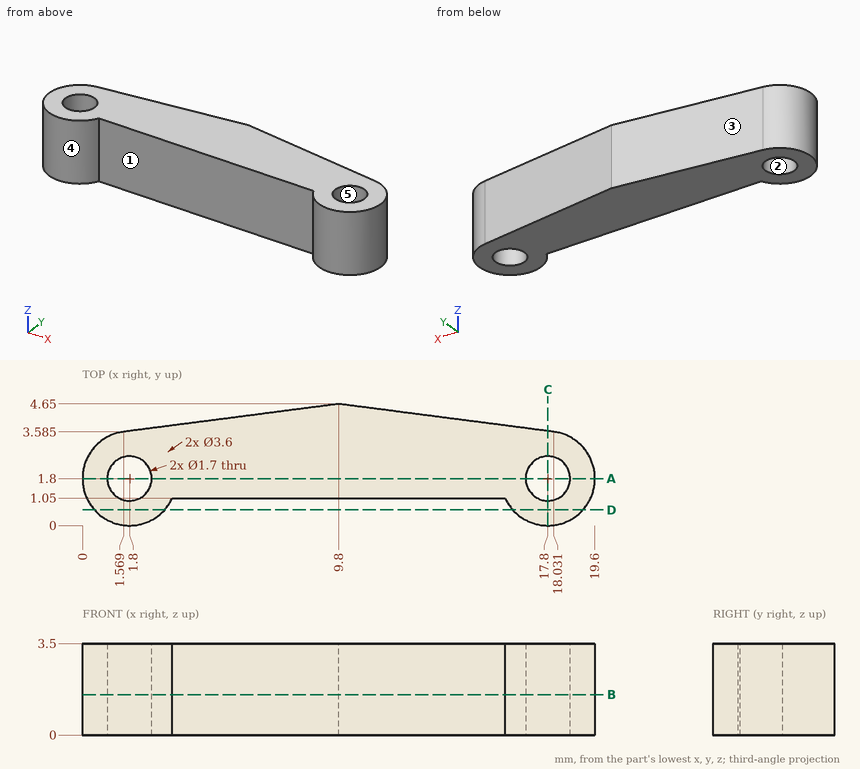
Geometry: see drawing. Coordinates: mm, zero at the bounding-box minimum. A direction names the side the tool comes from. Round coordinates to 2 decimals unless told otherwise and drop trailing zeros. Write each loop counter-clockwise with the first axis right and the second up, starting at its lowest first coordinate (ties: lowest second). Pieces come first, ordered by that corner, then holes.
1) Draft query along Y for the marked faces 3, 4 and 5. Return one class per face: pulls with the +Y half, pulls with the -Y half, needs draft (parallel to the pull), parting line crosses it, or undercut.
2) Cut plane C-C (x = 17.8). Return the cut outline in (y, z) (3 decimals).
3) Cut plane A-A (y = 1.8). Return the cut outline in (x, z).
4) Cut plane D-D (y = 0.6). Return the cut outline in (x, z), then the cut area to 3 significant figures.
5) Ray query, L1, parallel to X at y = 1.8, z = 1.85; L2, parallel to Y at x = 1.8, z = 1.5 (3 decimals). Return the intervals inside material, ascending.
6) Reachability of the marked faces 1 and 2 from +Z, -Z, +X, -X, +Y, -Y: full face, straight path, thin tool, end or side. Return the list, or none.
7) Contact query for flat-ended pins moving along their axis: P1, Ø1, axis at x = 15.5, z = 2.5, coming from the +Y side; P2, Ø1, axis at x = 7, z = 2.5, coming from the -Y side; P3, Ø1, axis at y = 1, z = 2.5, coming from the +X side (3 decimals). Output: stop coordinate, or through.
8) Cut plane B-B (z = 1.55). Count the separate pieces of the cut face and the enclosed holes in it, then the cut area to 3 significant figures.
Geometry says:
1. face 3: pulls with the +Y half
1. face 4: parting line crosses it
1. face 5: undercut
2. outline: (0, 0) - (0.95, 0) - (0.95, 3.5) - (0, 3.5) - close; (2.65, 0) - (3.615, 0) - (3.615, 3.5) - (2.65, 3.5) - close
3. outline: (0, 0) - (0.95, 0) - (0.95, 3.5) - (0, 3.5) - close; (2.65, 0) - (16.95, 0) - (16.95, 3.5) - (2.65, 3.5) - close; (18.65, 0) - (19.6, 0) - (19.6, 3.5) - (18.65, 3.5) - close
4. outline: (0.46, 0) - (3.14, 0) - (3.14, 3.5) - (0.46, 3.5) - close; (16.46, 0) - (19.14, 0) - (19.14, 3.5) - (16.46, 3.5) - close
4. area: 18.8 mm2
5. L1: x = 0 to 0.95, 2.65 to 16.95, 18.65 to 19.6
5. L2: y = 0 to 0.95, 2.65 to 3.615
6. face 1: +Z, -Z, -Y
6. face 2: +Z, -Z
7. P1: stops at y = 3.98
7. P2: stops at y = 1.05
7. P3: stops at x = 19.575
8. separate pieces: 1
8. enclosed holes: 2
8. area: 57.4 mm2
